```python
from build123d import *

# Parameters (mm, degrees)
SKETCH_2_W      = 100
SKETCH_2_H      = 100
SKETCH_2_R      = 2
SKETCH_2_W_2    = 50
SKETCH_2_H_2    = 50
EXTRUDE_1_DEPTH = 2.5
EXTRUDE_2_DEPTH = 82.5
EXTRUDE_3_DEPTH = 3
EXTRUDE_4_DEPTH = 35
EXTRUDE_5_DEPTH = 2


with BuildPart() as part:
    # 스케치2 → 보스-돌출1 (new, symmetric)
    with BuildSketch(Plane(origin=(0, 0, 0), x_dir=(1, 0, 0), z_dir=(0, 1, 0))):
        Rectangle(SKETCH_2_W, SKETCH_2_H)
        with Locations(Location((-44, 44, 0), (0, 0, 270))):
            Circle(SKETCH_2_R, mode=Mode.SUBTRACT)
        with Locations(Location((44, 44, 0), (0, 0, 270))):
            Circle(SKETCH_2_R, mode=Mode.SUBTRACT)
        with Locations(Location((-44, -44, 0), (0, 0, 270))):
            Circle(SKETCH_2_R, mode=Mode.SUBTRACT)
        with Locations(Location((44, -44, 0), (0, 0, 270))):
            Circle(SKETCH_2_R, mode=Mode.SUBTRACT)
        Rectangle(SKETCH_2_W_2, SKETCH_2_H_2, mode=Mode.SUBTRACT)
    extrude(amount=EXTRUDE_1_DEPTH, both=True)

    # 스케치3 → 보스-돌출2 (add, symmetric)
    with BuildSketch(Plane(origin=(0, 0, 0), x_dir=(0, 0, -1), z_dir=(1, 0, 0))):
        Polygon((-30.5, 0), (-30.5, 16), (-26.5, 16), (-26.5, 13), (-27.5, 13), (-27.5, 0), align=None)
        Polygon((27.5, 0), (30.5, 0), (30.5, 16), (26.5, 16), (26.5, 13), (27.5, 13), align=None)
    extrude(amount=EXTRUDE_2_DEPTH, both=True)

    # 스케치4 → 보스-돌출3 (add)
    with BuildSketch(Plane(origin=(82.5, 0, 0), x_dir=(0, 0, -1), z_dir=(1, 0, 0))):
        Polygon((-30.5, 16), (-25.5, 16), (-25.5, 4.5), (25.5, 4.5), (25.5, 16), (30.5, 16), (30.5, 0), (-30.5, 0), align=None)
    extrude(amount=EXTRUDE_3_DEPTH)

    # 스케치6 → 보스-돌출4 (add, symmetric)
    with BuildSketch(Plane.XY):
        Polygon((-20.75, 0), (-20.75, -21.5), (20.75, -21.5), (20.75, 0), (17.75, 0), (17.75, -18.5), (-17.75, -18.5), (-17.75, 0), align=None)
    extrude(amount=EXTRUDE_4_DEPTH, both=True)

    # 스케치7 → 보스-돌출5 (add)
    with BuildSketch(Plane.ZY.offset(82.5)):
        Polygon((27.5, 3.2), (-27.5, 3.2), (-27.5, 13), (-26.5, 13), (-26.5, 16), (-30.5, 16), (-30.5, 0), (30.5, 0), (30.5, 16), (26.5, 16), (26.5, 13), (27.5, 13), align=None)
    extrude(amount=EXTRUDE_5_DEPTH)


solid = part.part
```
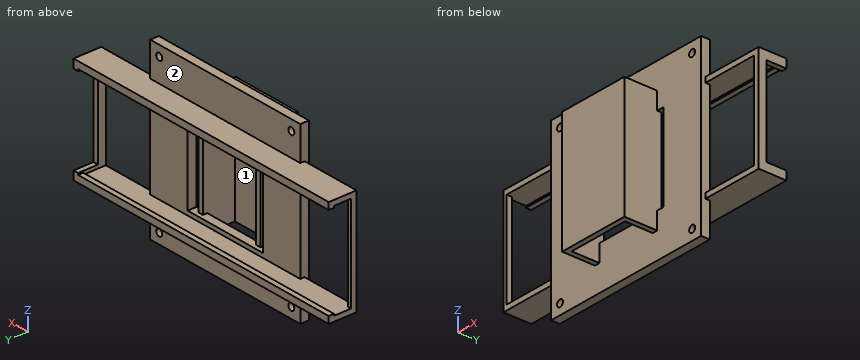
Here's how the part is built. I have some questions about the finished solid (model axes, mm). Face numbers are marked on the shaded views. Give positions to 0.01 mm unless a question says otherwise; leave off trailing zeros. Loops run counter-clockwise (first coordinate to the right, second up) from the corner with the lowest first, then second, coordinate; pieces in that order, holes last. Notation, with made-up numbers: M 54.25,56.5 L 84.25,56.5 A33 ccw 84.25,88.5 Z; hole C -7.5,51 d6. An arc over 180 degrees is marked long. Return JSON: item names as keys, results as strings.
Item 1: Imagine slicing it at D-D on z = -33. List the corners of the cut face in (x, y) for me, then the cut area to 4 significant figures.
A:
{"outline": "M -50,-2.5 L -20.75,-2.5 L -20.75,-21.5 L 20.75,-21.5 L 20.75,-2.5 L 50,-2.5 L 50,2.5 L -50,2.5 Z; hole M -17.75,-18.5 L 17.75,-18.5 L 17.75,-2.5 L -17.75,-2.5 Z", "area": "720.5 mm^2"}
Item 2: Thinking about a two-plate mould opening in X: for the marked faces 1 and 2, which applies, released by +X, released by -X, zero draft, split by the parting line, or undercut?
A:
{"face 1": "undercut", "face 2": "zero draft"}
Item 3: Imagine slicing it at C-C on y = -15. List the corners of the cut face in (x, z) for me.
A:
{"outline": "M -20.75,-35 L -17.75,-35 L -17.75,35 L -20.75,35 Z; M 17.75,-35 L 20.75,-35 L 20.75,35 L 17.75,35 Z"}
Item 4: Imagine slicing it at B-B on x = 52. List the corners of the cut face in (y, z) for me, then the cut area to 3 significant figures.
A:
{"outline": "M 0,-30.5 L 16,-30.5 L 16,-26.5 L 13,-26.5 L 13,-27.5 L 0,-27.5 Z; M 0,27.5 L 13,27.5 L 13,26.5 L 16,26.5 L 16,30.5 L 0,30.5 Z", "area": "102 mm^2"}
Item 5: Imagine slicing it at A-A on z = -44. List the corners of the cut face in (x, y) for me.
A:
{"outline": "M -50,-2.5 L -46,-2.5 L -46,2.5 L -50,2.5 Z; M -42,-2.5 L 42,-2.5 L 42,2.5 L -42,2.5 Z; M 46,-2.5 L 50,-2.5 L 50,2.5 L 46,2.5 Z"}
Item 6: Please list where these lines run through material, in increasing order: line 1 (X direction, y = 0, z = -44); line 2 (X direction, y = -4, z = -2.5); line 3 (Y direction, x = -5, z = 29).
A:
{"line 1": "x = -50 to -46, -42 to 42, 46 to 50", "line 2": "x = -20.75 to -17.75, 17.75 to 20.75", "line 3": "y = -21.5 to -18.5, -2.5 to 16"}
Item 7: I'm going to push flat-ended pins straight in: pin 1 Ø4.5 at (x, z) = (44, 44) entering from +Y; pin 2 Ø10.5 at (x, z) = (1, 5) entering from +Y; pin 3 Ø1.5 at (x, z) = (-19, 0.5) entering from +Y; pin 4 Ø10 at (x, z) = (-57.5, -11.5) entering from +Y. Where does each tip first touch, or does it pass through?
A:
{"pin 1": "stops at y = 2.5", "pin 2": "stops at y = -18.5", "pin 3": "stops at y = 0", "pin 4": "passes through"}
